Could you check a few things on this model? Use its own coordinates, in mm. Face numbers are marked on the shaded views. A direction names the side the tool comes from. Round coordinates to 2 decimals unless told otherwise and drop trailing zeros. Write each loop counter-clockwise with the first axis right and the second up, starting at its lowest first coordinate (ties: lowest second). Pieces come first, ordered by that corner, then holes. Notation, with made-up numbers: (-8, -29) - (25, -29) arc R17 cw to (25, -5) - close; hole circle Ø2 at (-19, 12). An arc over 180 degrees is marked (long way). Put each result on its own line as item: value.
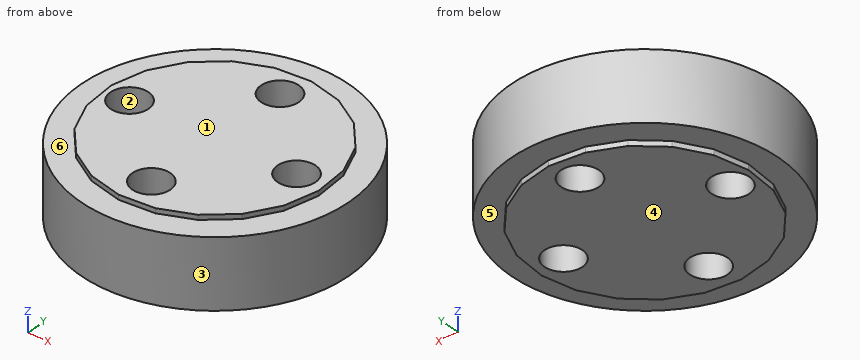
from build123d import *

# Parameters (mm, degrees)
F1_R          = 49.681019
F3_DEPTH      = 25.4
F4_DEPTH      = 27.178
F4_DEPTH_BACK = 2.032
F0_R          = 7.041454
F5_DEPTH      = 75.184
F5_DEPTH_BACK = 119.126


with BuildPart() as f3:
    # F1 (on Top) → F3 (new body)
    with BuildSketch(Plane.XY):
        Circle(F1_R)
    extrude(amount=F3_DEPTH)

    # F2 (on Top) → F4 (join, two sides)
    with BuildSketch(Plane.XY) as f4_sk:
        Polygon((-31.21903, 26.349589), (-37.833532, 15.412737), (-40.744625, 2.96718), (-39.66735, -9.768826), (-34.707159, -21.548591), (-26.349589, -31.21903), (-15.412737, -37.833532), (-2.96718, -40.744625), (9.768826, -39.66735), (21.548591, -34.707159), (31.21903, -26.349589), (37.833532, -15.412737), (40.744625, -2.96718), (39.66735, 9.768826), (34.707159, 21.548591), (26.349589, 31.21903), (15.412737, 37.833532), (2.96718, 40.744625), (-9.768826, 39.66735), (-21.548591, 34.707159), align=None)
    extrude(amount=F4_DEPTH)
    extrude(f4_sk.sketch, amount=-F4_DEPTH_BACK)

    # F0 (on Top) → F5 (cut, two sides)
    with BuildSketch(Plane.XY) as f5_sk:
        with Locations((0, 29.98014)):
            Circle(F0_R)
        with Locations((30.184653, 0)):
            Circle(F0_R)
        with Locations((0, -29.360153)):
            Circle(F0_R)
        with Locations((-31.631861, 0)):
            Circle(F0_R)
    extrude(amount=F5_DEPTH, mode=Mode.SUBTRACT)
    extrude(f5_sk.sketch, amount=-F5_DEPTH_BACK, mode=Mode.SUBTRACT)


solid = f3.part
(1) Imagine slicing it at A-A, the plane x = 29.5. List the corners of the cut face in (y, z) for me, then the cut area to 3 significant figures.
Values found:
outline: (-39.97, 0) - (-27.84, 0) - (-27.84, -2.03) - (-7.01, -2.03) - (-7.01, 27.18) - (-27.84, 27.18) - (-27.84, 25.4) - (-39.97, 25.4) - close; (7.01, -2.03) - (27.57, -2.03) - (27.57, 0) - (39.97, 0) - (39.97, 25.4) - (27.57, 25.4) - (27.57, 27.18) - (7.01, 27.18) - close
area: 1,830 mm^2
(2) I'm going to push flat-ended pins straight in: pin 1 (4 mm diameter, centred on x = -23.5, z = 2, fed in from +Y); pin 2 (1.5 mm diameter, centred on y = -27, z = 4, fed in from +X); pin 3 (12 mm diameter, centred on y = 36.5, z = 14, fed in from -X). Where does each tip first touch, or does it pass through?
Values found:
pin 1: stops at y = 44.79
pin 2: stops at x = 42.18
pin 3: stops at x = -39.22
(3) For the marked faces 4, 5 and 6, which set-ups out of +Z, -Z, +X, -X, +Y, -Y let a thin tool reach every point of the face, with its end or its side?
Values found:
face 4: -Z, +X, -X, +Y, -Y
face 5: -Z
face 6: +Z
(4) Imagine slicing it at B-B, the plane y = 0. List the corners of the cut face in (x, z) for me.
Values found:
outline: (-49.68, 0) - (-40.49, 0) - (-40.49, -2.03) - (-38.67, -2.03) - (-38.67, 27.18) - (-40.49, 27.18) - (-40.49, 25.4) - (-49.68, 25.4) - close; (-24.59, -2.03) - (23.14, -2.03) - (23.14, 27.18) - (-24.59, 27.18) - close; (37.23, -2.03) - (40.49, -2.03) - (40.49, 0) - (49.68, 0) - (49.68, 25.4) - (40.49, 25.4) - (40.49, 27.18) - (37.23, 27.18) - close
(5) If we mould it in two halves opening along X, with no side actions, what happens to the marked faces 1, 2 and 3? For each: pulls with the +X half, pulls with the -X half, needs draft (parallel to the pull), parting line crosses it, or undercut.
Values found:
face 1: needs draft
face 2: undercut
face 3: parting line crosses it
(6) Please list where these lines run through material, in increasing order: probe 1 along Y at (x, z) = (0, 18.5); probe 2 along X at (y, z) = (-5, 23.75); probe 3 along Y at (x, z) = (3, 23.5). Write a range as from..to.
Values found:
probe 1: y = -49.68..-36.4, -22.32..22.94, 37.02..49.68
probe 2: x = -49.43..-36.59, -26.67..25.23, 35.14..49.43
probe 3: y = -49.59..-35.73, -22.99..23.61, 36.35..49.59
(7) Imagine slicing it at C-C, the plane x = 0. List the corners of the cut face in (y, z) for me.
Values found:
outline: (-49.68, 0) - (-40.49, 0) - (-40.49, -2.03) - (-36.4, -2.03) - (-36.4, 27.18) - (-40.49, 27.18) - (-40.49, 25.4) - (-49.68, 25.4) - close; (-22.32, -2.03) - (22.94, -2.03) - (22.94, 27.18) - (-22.32, 27.18) - close; (37.02, -2.03) - (40.49, -2.03) - (40.49, 0) - (49.68, 0) - (49.68, 25.4) - (40.49, 25.4) - (40.49, 27.18) - (37.02, 27.18) - close
(8) Imagine slicing it at D-D, the plane z = 19. List the corners of the cut face in (x, y) for me, then the cut area to 3 significant figures.
Values found:
outline: circle Ø99.36 at (0, 0); hole circle Ø14.08 at (-31.63, 0); hole circle Ø14.08 at (0, -29.36); hole circle Ø14.08 at (0, 29.98); hole circle Ø14.08 at (30.18, 0)
area: 7,130 mm^2
